from build123d import *

# Parameters (mm, degrees)
SKETCH_2_W             = 500
SKETCH_2_H             = 150
SM_BASE_FLANGE_1_DEPTH = 4
SKETCH_7_R             = 7.5
CUT_EXTRUDE_1_DEPTH    = 10
CUT_EXTRUDE_2_DEPTH    = 10
SKETCH_9_W             = 500
SKETCH_9_H             = 70
EXTRUDE_1_DEPTH        = 4
SKETCH_11_W            = 294.318295345
SKETCH_11_H            = 76.206928483
CUT_EXTRUDE_3_DEPTH    = 10
SKETCH_12_R            = 14
CUT_EXTRUDE_4_DEPTH    = 10
SKETCH_13_R            = 1.65
CUT_EXTRUDE_5_DEPTH    = 10


# Sheet-metal steps are written as plain solids
with BuildPart() as part:
    # Sketch 2 → 基体-法兰1 (new body)
    with BuildSketch(Plane.XY):
        Rectangle(SKETCH_2_W, SKETCH_2_H)
    extrude(amount=-SM_BASE_FLANGE_1_DEPTH)

    # 草图7 → 切除-拉伸1 (cut)
    with BuildSketch(Plane.XY):
        with Locations((-50, 0)):
            Circle(SKETCH_7_R)
        with Locations((50, 0)):
            Circle(SKETCH_7_R)
    extrude(amount=-CUT_EXTRUDE_1_DEPTH, mode=Mode.SUBTRACT)

    # 草图8 → 切除-拉伸2 (cut)
    with BuildSketch(Plane.XY):
        Polygon((250, 45), (50, -75), (250, -75), align=None)
        Polygon((-250, -75), (-250, 45), (-50, -75), align=None)
    extrude(amount=-CUT_EXTRUDE_2_DEPTH, mode=Mode.SUBTRACT)

    # 草图9 → 凸台-拉伸1 (add)
    with BuildSketch(Plane(origin=(0, 0, -4), x_dir=(-1, 0, 0), z_dir=(0, 0, -1))):
        with Locations((0, 110)):
            Rectangle(SKETCH_9_W, SKETCH_9_H)
    extrude(amount=-EXTRUDE_1_DEPTH)

    # 草图11 → 切除-拉伸3 (cut)
    with BuildSketch(Plane(origin=(0, 0, -4), x_dir=(-1, 0, 0), z_dir=(0, 0, -1))):
        with Locations((38.825814339, -78.103464242)):
            Rectangle(SKETCH_11_W, SKETCH_11_H)
    extrude(amount=-CUT_EXTRUDE_3_DEPTH, mode=Mode.SUBTRACT)

    # 草图12 → 切除-拉伸4 (cut)
    with BuildSketch(Plane(origin=(0, 0, -4), x_dir=(-1, 0, 0), z_dir=(0, 0, -1))):
        with Locations((220, 70)):
            Circle(SKETCH_12_R)
    extrude(amount=-CUT_EXTRUDE_4_DEPTH, mode=Mode.SUBTRACT)

    # 草图13 → 切除-拉伸5 (cut)
    with BuildSketch(Plane(origin=(0, 0, -4), x_dir=(-1, 0, 0), z_dir=(0, 0, -1))):
        with Locations((220, 87.5)):
            Circle(SKETCH_13_R)
        with Locations((237.5, 70)):
            Circle(SKETCH_13_R)
        with Locations((220, 52.5)):
            Circle(SKETCH_13_R)
        with Locations((202.5, 70)):
            Circle(SKETCH_13_R)
    extrude(amount=-CUT_EXTRUDE_5_DEPTH, mode=Mode.SUBTRACT)


solid = part.part
Input: part model. Units: mm. Frame: model coordinates. Coordinates: 2 decimals unless noted, no trailing zeros. Order: outer loops, then holes, each group sorted by start corner. A loop starts at its lowest first (then second) coordinate and runs counter-clockwise, first axis right, second up.
1. Draft query along Y for faces 1 (the flat face through (-180, 3, -2)), 2 (the cylindrical face through (-42.846, 2.253, -1.972)), 3 (the flat face through (3, 54, 0)). Return one class per face: +Y half, -Y half, draft (parallel to the pull), parting line (faces both ways), or undercut.
Checked values:
face 1: -Y half
face 2: undercut
face 3: draft
2. Cut plane C-C, the plane y = 0. Return loops of the section in (x, z), plus the area to 3 significant figures.
Checked values:
outline: (-175, -4) - (-57.5, -4) - (-57.5, 0) - (-175, 0) - close; (-42.5, -4) - (42.5, -4) - (42.5, 0) - (-42.5, 0) - close; (57.5, -4) - (175, -4) - (175, 0) - (57.5, 0) - close
area: 1,280 mm2
3. Cut plane A-A, the plane z = -2.9. Return loops of the section in (x, y).
Checked values:
outline: (-250, 45) - (-108.33, -40) - (108.33, -40) - (250, 45) - (250, 145) - (-250, 145) - close; hole circle Ø3.3 at (-237.5, 70); hole circle Ø28 at (-220, 70); hole circle Ø3.3 at (-220, 52.5); hole circle Ø3.3 at (-220, 87.5); hole circle Ø3.3 at (-202.5, 70); hole circle Ø15 at (-50, 0); hole circle Ø15 at (50, 0)
4. Ray query, line 1 along Y through (x, z) = (50, -3.8); line 2 along Y through (x, z) = (-220, -2.5); line 3 along X through (y, z) = (4, -0.2). Return the intervals inside material, ascending.
Checked values:
line 1: y = -40 to -7.5, 7.5 to 145
line 2: y = 27 to 50.85, 54.15 to 56, 84 to 85.85, 89.15 to 145
line 3: x = -181.67 to -56.34, -43.66 to 43.66, 56.34 to 181.67
5. Cut plane D-D, the plane x = -182.5. Return loops of the section in (y, z).
Checked values:
outline: (4.5, -4) - (145, -4) - (145, 0) - (4.5, 0) - close
6. Contact query for a flat-ended pin moving along its axis: P1, Ø13.5, axis at x = 50, y = 0, coming from the -Z side. Output: stop coordinate, or through.
Checked values:
P1: passes through
7. Cut plane B-B, the plane x = -50. Return loops of the section in (y, z), plus the area to 3 significant figures.
Checked values:
outline: (-40, -4) - (-7.5, -4) - (-7.5, 0) - (-40, 0) - close; (7.5, -4) - (145, -4) - (145, 0) - (7.5, 0) - close
area: 680 mm2
